Could you check a few things on this model? Use its own coordinates, in mm. Face numbers are marked on the shaded views. A direction names the side the tool comes from. Give positions to 0.01 mm unless a question says otherwise; leave off trailing zeros. Loops run counter-clockwise (first coordinate to the right, second up) from the corner with the lowest first, then second, coordinate; pieces in that order, holes last. Notation, with made-up numbers: (-34, 87) - (14, 87) arc R36 cw to (14, 126) - close; hole circle Ø6 at (34, 2). An arc over 180 degrees is marked (long way). Write each question's results on one line, items separated by ' | '. Start each with the question number.
1) If I drill on probe 1 along X at (y, z) = (-16.85, 11); probe 2 along Y at (x, z) = (32, 5.75); probe 3 along Z at (x, y) = (59.5, -1), over which ranges is the centre line in solid material (lowest first)? Write a range as [from, to].
2) I want a section at B-B, the plane z = 17.5. Write out the boundary of the cut face in (x, y).
3) I want a section at D-D, the plane z = 12.5. Write out the boundary of the cut face in (x, y).
4) I want a section at C-C, the plane y = 0. Write out the boundary of the cut face in (x, z), and give its area (3 significant figures).
5) If we mould it in two halves opening along Y, with no side actions, what happens to the marked faces 1, 2, 3 and 4? For each: +Y half, -Y half, draft (parallel to the pull), parting line (faces both ways), or undercut.
6) On a 3-axis mill with a long thin cutter (end or side, diameter ignored), from which of +Z, -Z, +X, -X, +Y, -Y can I reach the whole of each face in a straight line? I mean the marked faces 5 and 6. Say none if no direction works.
7) I want a section at A-A, the plane x = 57.5. Write out the boundary of the cut face in (y, z).
8) I'm going to push flat-ended pins straight in: pin 1 (1 mm diameter, centred on x = 64.5, z = 2, fed in from -Y); pin 2 (2 mm diameter, centred on x = 22.5, y = 5, fed in from +Z); pin 3 (4.5 mm diameter, centred on x = 26.5, z = 11, fed in from -Y). Where does each tip first touch, or does it pass through?
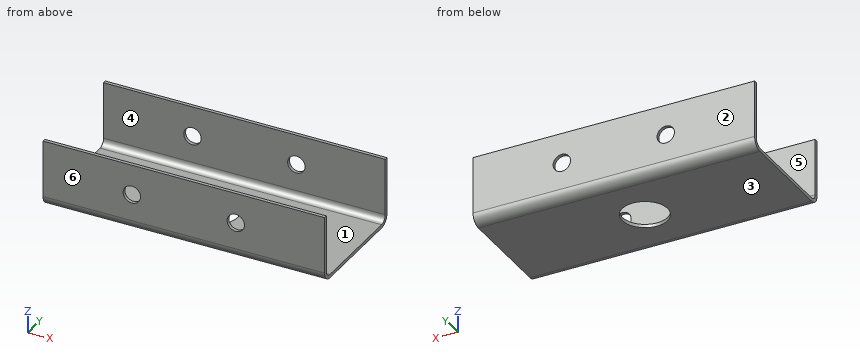
from build123d import *

# Parameters (mm, degrees)
BASE_FLANGE1_DEPTH = 84
SKETCH14_R         = 2.6
CUT_EXTRUDE1_DEPTH = 94.171884171
SKETCH15_R         = 6.75
CUT_EXTRUDE2_DEPTH = 89.103632161


# Sheet-metal steps are written as plain solids
with BuildPart() as part:
    # Sketch3 → Base-Flange1 (new body)
    with BuildSketch(Plane(origin=(0, 0, 0), x_dir=(0, 0, -1), z_dir=(1, 0, 0))):
        with BuildLine():
            Line((-20, 17.5), (-3, 17.5))
            ThreePointArc((-3, 17.5), (-0.878679656, 16.621320344), (0, 14.5))
            Line((0, 14.5), (0, -14.5))
            ThreePointArc((0, -14.5), (-0.878679656, -16.621320344), (-3, -17.5))
            Line((-3, -17.5), (-20, -17.5))
            Line((-20, -17.5), (-20, -16.5))
            Line((-20, -16.5), (-3, -16.5))
            ThreePointArc((-3, -16.5), (-1.585786438, -15.914213562), (-1, -14.5))
            Line((-1, -14.5), (-1, 14.5))
            ThreePointArc((-1, 14.5), (-1.585786438, 15.914213562), (-3, 16.5))
            Line((-3, 16.5), (-20, 16.5))
            Line((-20, 16.5), (-20, 17.5))
        make_face()
    extrude(amount=BASE_FLANGE1_DEPTH)

    # Sketch14 → Cut-Extrude1 (cut, through all)
    with BuildSketch(Plane(origin=(0, 17.5, 0), x_dir=(1, 0, 0), z_dir=(0, 1, 0))):
        with Locations(Location((26.5, -11, 0), (0, 0, 270))):
            Circle(SKETCH14_R)
        with Locations(Location((57.5, -11, 0), (0, 0, 270))):
            Circle(SKETCH14_R)
    extrude(amount=-CUT_EXTRUDE1_DEPTH, mode=Mode.SUBTRACT)

    # Sketch15 → Cut-Extrude2 (cut, through all)
    with BuildSketch(Plane(origin=(0, 0, 0), x_dir=(-1, 0, 0), z_dir=(0, 0, -1))):
        with Locations((-42, 0)):
            Circle(SKETCH15_R)
    extrude(amount=-CUT_EXTRUDE2_DEPTH, mode=Mode.SUBTRACT)


solid = part.part
Answers:
1) probe 1: x = [0, 23.9], [29.1, 54.9], [60.1, 84] | probe 2: y = [-17.5, -16.5], [16.5, 17.5] | probe 3: z = [0, 1]
2) outline: (0, -17.5) - (84, -17.5) - (84, -16.5) - (0, -16.5) - close; (0, 16.5) - (84, 16.5) - (84, 17.5) - (0, 17.5) - close
3) outline: (0, -17.5) - (24.38, -17.5) - (24.38, -16.5) - (0, -16.5) - close; (0, 16.5) - (24.38, 16.5) - (24.38, 17.5) - (0, 17.5) - close; (28.62, -17.5) - (55.38, -17.5) - (55.38, -16.5) - (28.62, -16.5) - close; (28.62, 16.5) - (55.38, 16.5) - (55.38, 17.5) - (28.62, 17.5) - close; (59.62, -17.5) - (84, -17.5) - (84, -16.5) - (59.62, -16.5) - close; (59.62, 16.5) - (84, 16.5) - (84, 17.5) - (59.62, 17.5) - close
4) outline: (0, 0) - (35.25, 0) - (35.25, 1) - (0, 1) - close; (48.75, 0) - (84, 0) - (84, 1) - (48.75, 1) - close | area: 70.5 mm2
5) face 1: undercut | face 2: +Y half | face 3: draft | face 4: undercut
6) face 5: +Z, +X, -X | face 6: +Z, -Z, +X, -X, -Y
7) outline: (-17.5, 3) arc R3 ccw to (-14.5, 0) - (14.5, 0) arc R3 ccw to (17.5, 3) - (17.5, 8.4) - (16.5, 8.4) - (16.5, 3) arc R2 cw to (14.5, 1) - (-14.5, 1) arc R2 cw to (-16.5, 3) - (-16.5, 8.4) - (-17.5, 8.4) - close; (-17.5, 13.6) - (-16.5, 13.6) - (-16.5, 20) - (-17.5, 20) - close; (16.5, 13.6) - (17.5, 13.6) - (17.5, 20) - (16.5, 20) - close
8) pin 1: stops at y = -17.46 | pin 2: stops at z = 1 | pin 3: passes through
